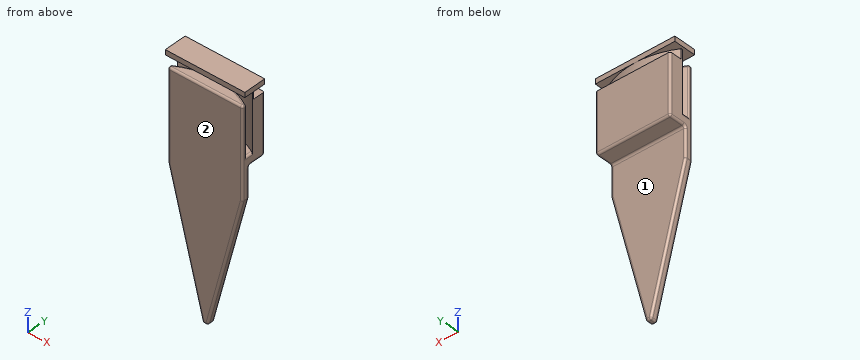
Autodesk Fusion 360 part; units mm, degrees
sketch "Sketch1" plane through (0, 0, 0) normal (0, 0, 1) x (1, 0, 0)
  line L0 (0, 5) -> (15, 5)
  line L1 (15, 5) -> (15, 0)
  line L2 (15, 0) -> (0, 0)
  line L3 (0, 0) -> (0, 5)
  arc A0 (15, 0.75) -> (0, 0.75) centre (7.5, -11.5062) ccw
  arc A1 (15, 2.25) -> (0, 2.25) centre (7.5, -10.8125) ccw
  line L4 (0, 4.25) -> (15, 4.25) construction
  line L5 (0, 1.5) -> (15, 1.5)
  arc A2 (15, 2.5) -> (0, 2.5) centre (7.5, -10.5625) ccw
  dimension "d1" = 1.5
  dimension "d2" = 1.5
  dimension "d3" = 0.75
  dimension "d4" = 15
  dimension "d5" = 5
  dimension "d9" = 0.75
  dimension "d14" = 1.5
  dimension "d25" = 0.25
  dimension "d26" = 0.25
extrude "Extrude1" add sketch "Sketch1" against normal blind 2
extrude "Extrude2" add sketch "Sketch1" along normal blind 10 contours L0 L1 L3 A2 | L1 L3 A1 A2 | L1 L2 L3 A0 L5 | A0 L5
extrude "Extrude3" add sketch "Sketch1" against normal blind 35 contours L3 A0 L5 | L1 A0 L5 | L1 L2 L3 A0 L5
extrude "Extrude4" add sketch "Sketch1" along normal blind 12 and the other way blind -10 contours L1 L3 A1 A2
sketch "Sketch2" plane through (0, 0, 0) normal (0, -1, 0) x (1, 0, 0)
  line L0 (15, -35) -> (15, 10)
  line L1 (15, 10) -> (0, 10)
  line L2 (0, 10) -> (0, -35)
  line L3 (0, -35) -> (15, -35)
  line L4 (-0.5, 13) -> (15.5, 13)
  line L5 (15.5, 13) -> (15.5, 12)
  line L6 (15.5, 12) -> (-0.5, 12)
  line L7 (-0.5, 12) -> (-0.5, 13)
  dimension "d33" = 1
extrude "Extrude5" add sketch "Sketch2" against normal blind 4.5 contours L4 L5 L6 L7
chamfer "Chamfer1" distance 7 distance2 27 1 edges at (15, 0.75, -35) measured on face at (5, 1, -35)
chamfer "Chamfer2" distance 7 distance2 27 1 edges at (0, 0.75, -35) measured on face at (5.3333, 0.5, -35)
fillet "Fillet2" radius 0.4 28 edges at (11.5, 1.5, -21.5) (7.5, 1.5, -35) (3.5, 1.5, -21.5) (3.5, 0, -21.5) (11.5, 0, -21.5) (7.5, 0, -35) (8, 0.75, -35) (7, 0.75, -35) (15, 3.25, -2) (15, 0, 1) (15, 0.75, -8) (15, 1.5, -5) (15, 5, 4) (7.5, 5, -2) (7.5, 1.5, -2) (0, 5, 4) (0, 3.25, -2) (0, 1.5, -5) (0, 0.75, -8) (0, 0, 1) (7.5, 2.8627, 10) (15, 0.375, 10) (0, 0.375, 10) (15, 0.75, 5) (15, 1.5, 0) (0, 0.75, 5) (0, 1.5, 0) (7.5, 0, 10)
equation "d1 = d2"
equation "d26 = d25"
The listing builds one solid part. Answer for the finished solid, in the listing's coordinates (mm). Face numbers are marked on the shaded views. A direction names the side the tool comes from. Give positions to 0.01 mm unless a question says otherwise; leave off trailing zeros. Write each loop counter-clockwise with the first axis right and the second up, starting at its lowest first coordinate (ties: lowest second). Pieces come first, ordered by that corner, then holes. Notation, with made-up numbers: (36, 30) -> (89, 30) arc R32 ccw to (89, 66) -> close; hole circle Ø10 at (19, 6.5). An arc over 180 degrees is marked (long way). Use a Markdown table: item, result.
(1) For the marked faces 1 and 2, determine the directions among +Z, -Z, +X, -X, +Y, -Y from which every point of the face is accessible in a straight line to the end or side of a thin tool.
Return value:
| item | result |
|---|---|
| face 1 | -Z, +X, -X, +Y |
| face 2 | +Z, -Z, +X, -X, -Y |
(2) Flat-ended cylindrical pins translate along their axes: P1, Ø1, axis at y = 1.5, z = 0, coming from the -X side; P2, Ø2, axis at y = 1, z = -20.5, coming from the -X side; P3, Ø7, axis at x = 10, z = -11, coming from the +Y side. Find the tip coordinate at first contact, or state that the pin passes through.
Return value:
| item | result |
|---|---|
| P1 | x = 0 |
| P2 | x = 2.98 |
| P3 | y = 1.5 |
(3) Section B-B, the plane y = 3.4 is taken. Determine the outline of the cut face in (x, z), then the cut area to 3 significant figures.
Return value:
| item | result |
|---|---|
| outline | (-0.5, 12) -> (1.85, 12) -> (1.85, 10) -> (0, 10) -> (0, -1.6) arc R0.4 ccw to (0.4, -2) -> (14.6, -2) arc R0.4 ccw to (15, -1.6) -> (15, 10) -> (13.15, 10) -> (13.15, 12) -> (15.5, 12) -> (15.5, 13) -> (-0.5, 13) -> close; hole (2.51, 0) -> (12.49, 0) -> (12.49, 12) -> (2.51, 12) -> close |
| area | 98.8 mm2 |
(4) Find the intervals of material crossed by probe 1 along Z at (x, y) = (2.5, 3.9); probe 2 along Z at (x, y) = (9, 4.05); probe 3 along Y at (x, z) = (3, -16), in increasing order. Write a range as from..to.
Return value:
| item | result |
|---|---|
| probe 1 | -2..10, 12..13 |
| probe 2 | -2..0, 12..13 |
| probe 3 | 0..1.5 |
